Job drawing, mm, ordinate dimensions from the low corner. One solid piece. A direction names the side the tool comes from. Round coordinates to 2 decimals unless told otherwise and drop trailing zeros. Loops run counter-clockwise (first coordinate to the right, second up) from the corner with the lowest first, then second, coordinate; pieces in that order, holes last.
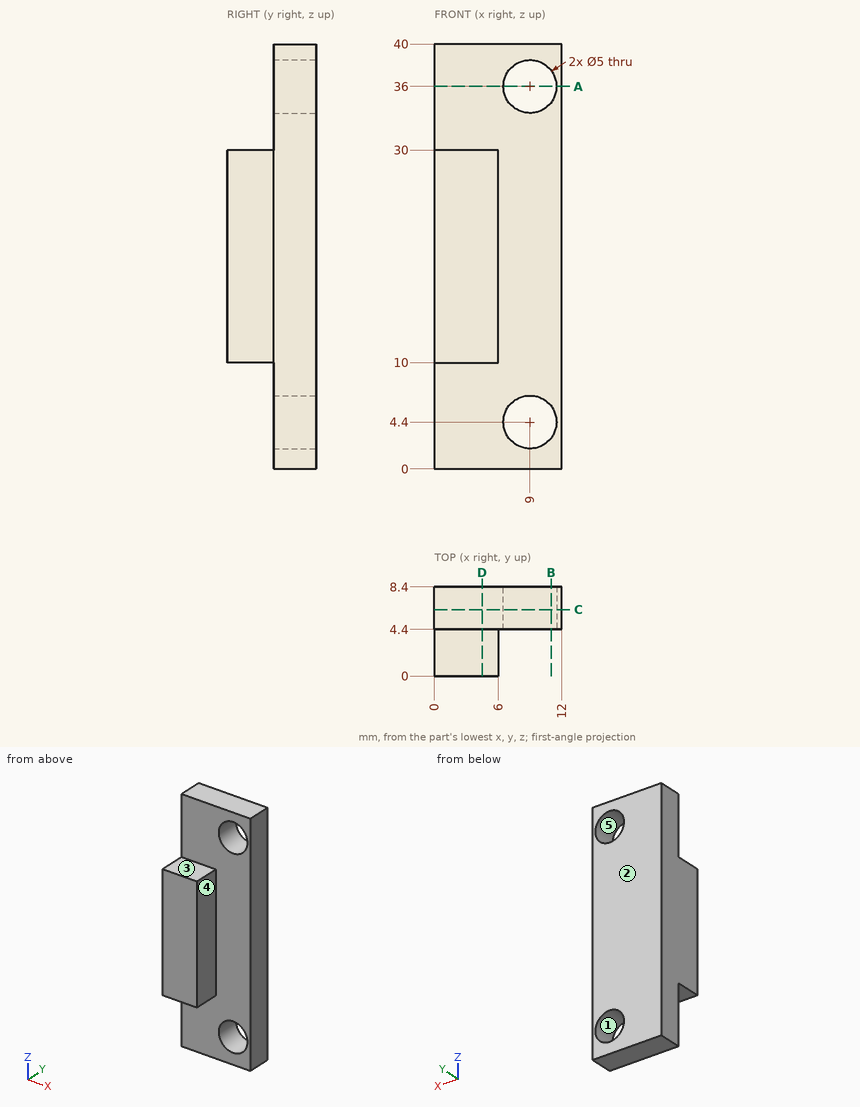
Item 1: Two-plate mould, pull along Z, no slides. Class the marked faces 1, 2 and 3: released by +Z, released by -Z, zero draft, split by the parting line, or undercut.
Answers follow:
face 1: undercut
face 2: zero draft
face 3: released by +Z
Item 2: Probe line 1 (Z direction, x = 9, y = 5.5); line 2 (X direction, y = 6.3, z = 4.4); line 3 (Z direction, x = 10.5, y = 4.5). List the from-to ranges inside material, lowest first.
Answers follow:
line 1: z = 0 to 1.9, 6.9 to 33.5, 38.5 to 40
line 2: x = 0 to 6.5, 11.5 to 12
line 3: z = 0 to 2.4, 6.4 to 34, 38 to 40
Item 3: Cut at A-A, the plane z = 36. Give the cut face in (x, y), plus the area to 3 significant figures.
Answers follow:
outline: (0, 4.4) - (6.5, 4.4) - (6.5, 8.4) - (0, 8.4) - close; (11.5, 4.4) - (12, 4.4) - (12, 8.4) - (11.5, 8.4) - close
area: 28.0 mm2
Item 4: Flat gauge pins, fed straight in: P1, Ø3.5, axis at y = 1, z = 19.5, coming from the +X side; P2, Ø1.3, axis at x = 2, y = 3, coming from the -Z side. Where does each tip first touch, or does it go through?
Answers follow:
P1: stops at x = 6
P2: stops at z = 10
Item 5: Cut at C-C, the plane y = 6.25. Give the cut face in (x, z), plus the area to 3 significant figures.
Answers follow:
outline: (0, 0) - (12, 0) - (12, 40) - (0, 40) - close; hole circle Ø5 at (9, 4.4); hole circle Ø5 at (9, 36)
area: 441 mm2
Item 6: 3-axis set-ups, long thin cutter, end or side, ignore diameter. For the marked faces 4 and 5: which of +Z, -Z, +X, -X, +Y, -Y reach the whole face in a straight line?
Answers follow:
face 4: +Z, -Z, +X, -Y
face 5: +Y, -Y
Item 7: Cut at D-D, the plane x = 4.5. Give the cut face in (y, z).
Answers follow:
outline: (0, 10) - (4.4, 10) - (4.4, 0) - (8.4, 0) - (8.4, 40) - (4.4, 40) - (4.4, 30) - (0, 30) - close
Item 8: Cut at B-B, the plane x = 11. Give the cut face in (y, z).
Answers follow:
outline: (4.4, 0) - (8.4, 0) - (8.4, 2.9) - (4.4, 2.9) - close; (4.4, 5.9) - (8.4, 5.9) - (8.4, 34.5) - (4.4, 34.5) - close; (4.4, 37.5) - (8.4, 37.5) - (8.4, 40) - (4.4, 40) - close
